The figure shows three views and two pictorial views of one solid part (mm, origin at its lowest corner). Answer the questions. A direction names the side the tool comes from. Give positions to 0.01 mm unless a question says otherwise; leave off trailing zeros. Write each loop counter-clockwise with the first axis right and the second up, starting at its lowest first coordinate (ties: lowest second). Pieces come first, ordered by that corner, then holes. Notation, with made-up numbers: (22.25, 45) -> (68.25, 45) arc R27 ccw to (68.25, 63) -> close; hole circle Ø5 at (84, 24.25). An arc over 180 degrees is marked (long way). Write item = value, one per line. Start each with the question number.
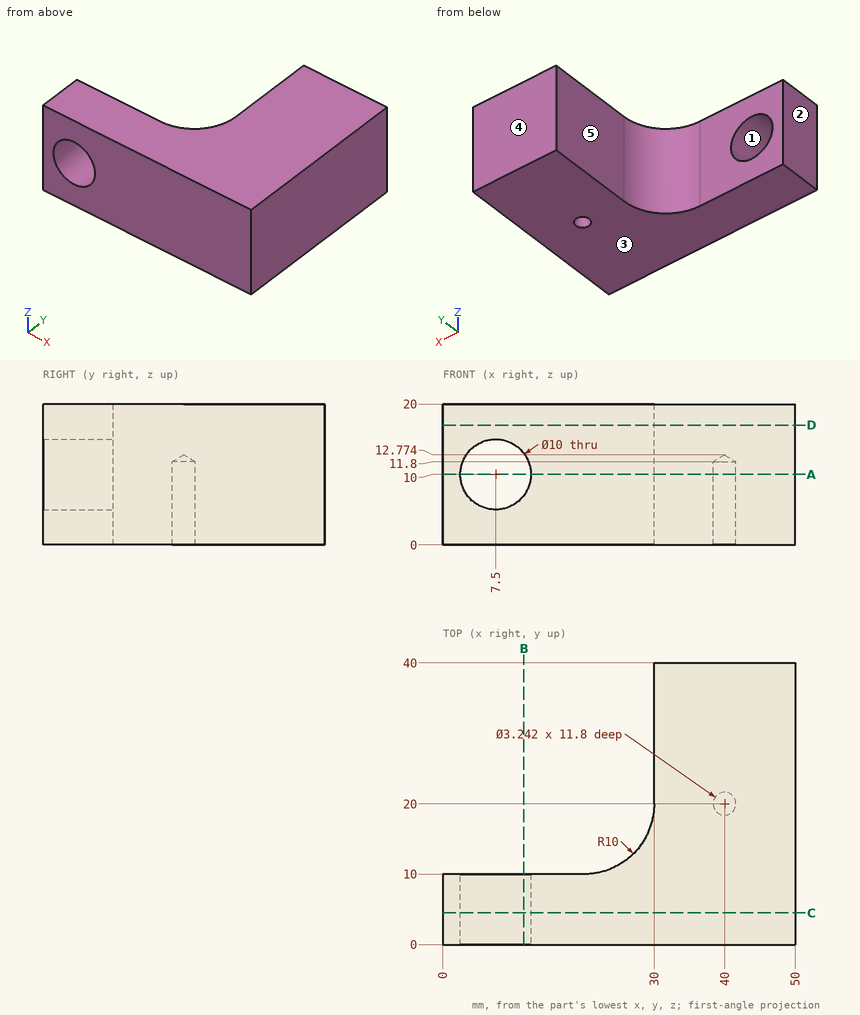
(1) Find the intervals of material crossed by line 1 along X through (y, z) = (20, 3.5); line 2 along X through (y, z) = (8.25, 10); line 3 along Y through (x, z) = (13, 14.75), in increasing order.
(2) A cutting plane is placed at D-D, the plane z = 17. Write down the section's boundary in (x, y).
(3) A cutting plane is placed at C-C, the plane y = 4.5. Write down the section's boundary in (x, z).
(4) A cutting plane is placed at A-A, the plane z = 10. Write down the section's boundary in (x, y).
(5) For the marked faces 4 and 5, determine the directions among +Z, -Z, +X, -X, +Y, -Y from which every point of the face is accessible in a straight line to the end or side of a thin tool.
(6) This flat-tipped pin is pushed along its axis until it touches: pin 1 (5 mm diameter, centred on y = 16, z = 13, fed in from -X). Where does it stop, or does it pass through?
(7) Determine the mould class of the marked faces 1, 2 and 3 for opening direction Z: pulls with the +Z half, pulls with the -Z half, needs draft (parallel to the pull), parting line crosses it, or undercut.
(8) A cutting plane is placed at B-B, the plane x = 11.5. Write down the section's boundary in (y, z), then the cut area to 3 significant figures.
Results list:
q1.line_1 = 30 to 38.38, 41.62 to 50
q1.line_2 = 0 to 2.5, 12.5 to 50
q1.line_3 = 0 to 10
q2.outline = (0, 0) -> (50, 0) -> (50, 40) -> (30, 40) -> (30, 20) arc R10 cw to (20, 10) -> (0, 10) -> close
q3.outline = (0, 0) -> (50, 0) -> (50, 20) -> (0, 20) -> close; hole circle Ø10 at (7.5, 10)
q4.outline = (0, 0) -> (2.5, 0) -> (2.5, 10) -> (0, 10) -> close; (12.5, 0) -> (50, 0) -> (50, 40) -> (30, 40) -> (30, 20) arc R10 cw to (20, 10) -> (12.5, 10) -> close; hole circle Ø3.24 at (40, 20)
q5.face_4 = +Z, -Z, +X, -X, +Y
q5.face_5 = +Z, -Z, -X, +Y
q6.pin_1 = 27.6
q7.face_1 = undercut
q7.face_2 = needs draft
q7.face_3 = pulls with the -Z half
q8.outline = (0, 0) -> (10, 0) -> (10, 7) -> (0, 7) -> close; (0, 13) -> (10, 13) -> (10, 20) -> (0, 20) -> close
q8.area = 140 mm²
